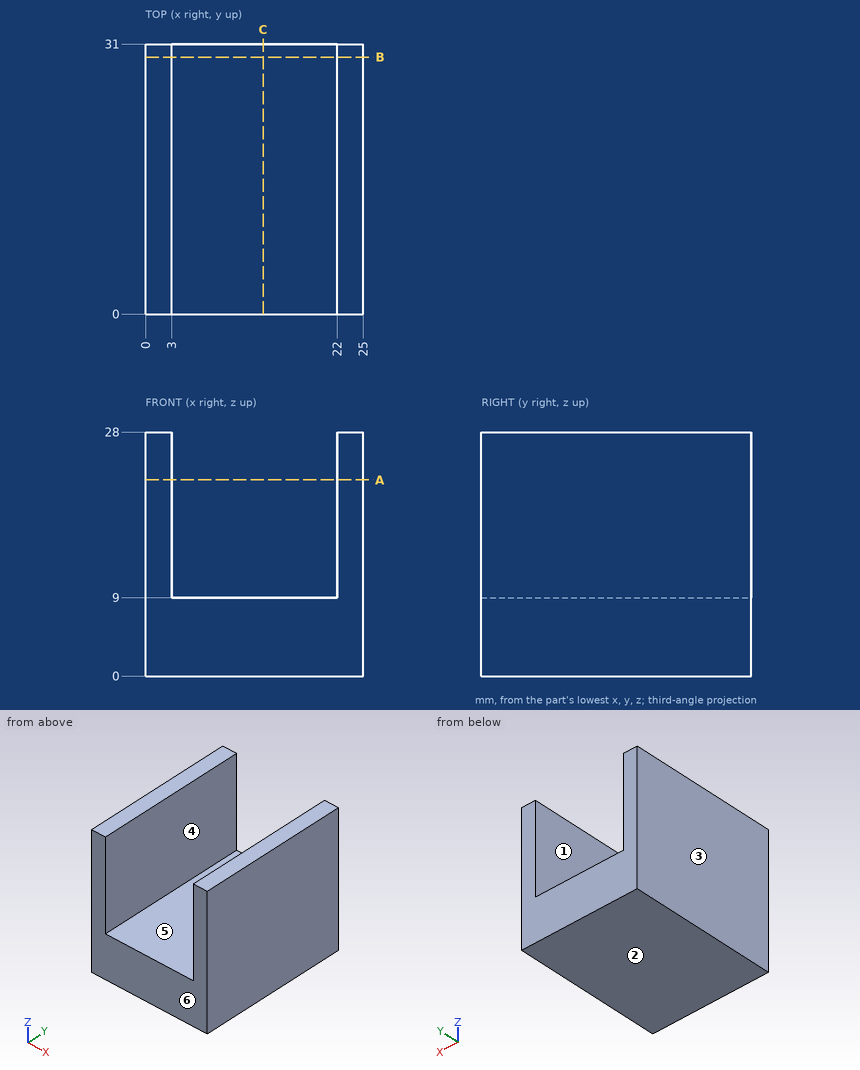
Part print with two shaded views. Sizes in mm from the minimum x, y, z corner. A direction names the side the tool comes from. Round coordinates to 2 decimals unless told otherwise and drop trailing zeros. Write each loop counter-clockwise with the first axis right and the second up, starting at its lowest first coordinate (ties: lowest second). Pieces come first, ordered by that corner, then holes. Notation, with made-up numbers: (5, -38) -> (20, -38) arc R29 cw to (20, -16) -> close; hole circle Ø5 at (77, 70). An arc over 180 degrees is marked (long way). Put each result on its own line as item: value.
Item 1: Two-plate mould, pull along X, no slides. Class the marked faces 1, 2, 3 and 4: pulls with the +X half, pulls with the -X half, needs draft (parallel to the pull), parting line crosses it, or undercut.
Here are the results:
face 1: undercut
face 2: needs draft
face 3: pulls with the -X half
face 4: undercut
Item 2: Slice it at A-A, the plane z = 22.5. Give the cut face in (x, y).
Here are the results:
outline: (0, 0) -> (3, 0) -> (3, 31) -> (0, 31) -> close; (22, 0) -> (25, 0) -> (25, 31) -> (22, 31) -> close
Item 3: Tool access for the marked faces 5 and 6: list every direction of +Z, -Z, +X, -X, +Y, -Y with a clear straight run to the whole face (end or side of a thin tool).
Here are the results:
face 5: +Z, +Y, -Y
face 6: +Z, -Z, +X, -X, -Y
Item 4: Flat gauge pins, fed straight in: P1, Ø6, axis at y = 23, z = 23.5, coming from the -X side; P2, Ø9.5, axis at x = 14, y = 19.5, coming from the +Z side. Where does each tip first touch, or does it go through?
Here are the results:
P1: stops at x = 0
P2: stops at z = 9
Item 5: Slice it at C-C, the plane x = 13.5. Give the cut face in (y, z).
Here are the results:
outline: (0, 0) -> (31, 0) -> (31, 9) -> (0, 9) -> close
Item 6: Wall check: probe 1 along X at (y, z) = (27.5, 23.5); probe 2 along Z at (x, y) = (8.75, 19.5). Give the ranges that are in metal, low to high. Write a range as from..to.
Here are the results:
probe 1: x = 0..3, 22..25
probe 2: z = 0..9
Item 7: Slice it at B-B, the plane y = 29.5. Give the cut face in (x, z).
Here are the results:
outline: (0, 0) -> (25, 0) -> (25, 28) -> (22, 28) -> (22, 9) -> (3, 9) -> (3, 28) -> (0, 28) -> close
